Autodesk Inventor part; units mm, degrees
ref_plane "YZ Plane" through (0, 0, 0) normal (1, 0, 0) x (0, 1, 0)
ref_plane "XZ Plane" through (0, 0, 0) normal (0, 1, 0) x (-1, 0, 0)
ref_plane "XY Plane" through (0, 0, 0) normal (0, 0, 1) x (1, 0, 0)
sketch "Sketch1" plane through (0, 0, 0) normal (0, 0, 1) x (1, 0, 0)
  line L0 (-110, -113.5) -> (110, -113.5)
  line L1 (110, -113.5) -> (110, 113.5)
  line L2 (110, 113.5) -> (-110, 113.5)
  line L3 (-110, 113.5) -> (-110, -113.5)
  line L4 (-110, -113.5) -> (110, 113.5) construction
  line L5 (110, -113.5) -> (-110, 113.5) construction
  point P0 (0, 0)
  dimension "d0" = 220
  dimension "d1" = 227
extrude "Extrusion1" add sketch "Sketch1" along normal blind 8
sketch "Sketch2" plane through (0, 0, 8) normal (0, 0, 1) x (1, 0, 0)
  line L0 (-107.55, -111.05) -> (107.55, -111.05)
  line L1 (107.55, -111.05) -> (107.55, 111.05)
  line L2 (107.55, 111.05) -> (-107.55, 111.05)
  line L3 (-107.55, 111.05) -> (-107.55, -111.05)
  line L4 (-107.55, -111.05) -> (107.55, 111.05) construction
  line L5 (107.55, -111.05) -> (-107.55, 111.05) construction
  point P0 (0, 0)
  dimension "d4" = 215.1
  dimension "d5" = 222.1
extrude "Extrusion2" cut sketch "Sketch2" against normal blind 1.6
sketch "Sketch3" plane through (0, 0, 6.4) normal (0, 0, 1) x (1, 0, 0)
  line L0 (-105, -108.5) -> (105, -108.5)
  line L1 (105, -108.5) -> (105, 108.5)
  line L2 (105, 108.5) -> (-105, 108.5)
  line L3 (-105, 108.5) -> (-105, -108.5)
  line L4 (-105, -108.5) -> (105, 108.5) construction
  line L5 (105, -108.5) -> (-105, 108.5) construction
  point P0 (0, 0)
  dimension "d8" = 210
  dimension "d9" = 217
extrude "Extrusion3" cut sketch "Sketch3" against normal blind 3.5
fillet "Fillet1" radius 2 8 edges at (-107.55, -111.05, 7.2) (-110, -113.5, 4) (110, -113.5, 4) (107.55, -111.05, 7.2) (110, 113.5, 4) (107.55, 111.05, 7.2) (-110, 113.5, 4) (-107.55, 111.05, 7.2)
sketch "Sketch4" plane through (0, 0, 2.9) normal (0, 0, 1) x (1, 0, 0)
  circle A0 centre (-103.9, 107.4) radius 5
  circle A1 centre (-103.9, -107.4) radius 5
  line L0 (-105.55, 111.05) -> (105.55, 111.05)
  circle A2 centre (103.9, 107.4) radius 5
  line L1 (107.55, 109.05) -> (107.55, -109.05)
  circle A3 centre (103.9, -107.4) radius 5
  line L2 (-107.55, -109.05) -> (-107.55, 109.05)
  point P0 (0, 0)
  dimension "d13" = 10
  dimension "d14" = 10
  dimension "d15" = 214.8
  dimension "d16" = 3.65
  dimension "d17" = 10
  dimension "d18" = 207.8
  dimension "d19" = 3.65
  dimension "d20" = 10
  dimension "d21" = 3.65
  dimension "d22" = 214.8
  dimension "d23" = 207.8
  dimension "d24" = 3.65
extrude "Extrusion4" add sketch "Sketch4" along normal blind 3.5
sketch "Sketch5" plane through (0, 0, 6.4) normal (0, 0, 1) x (1, 0, 0)
  arc A0 (-105, 102.5225) -> (-99.0225, 108.5) centre (-103.9, 107.4) ccw
  circle A1 centre (-103.9, 107.4) radius 1.4
  arc A2 (99.0225, 108.5) -> (105, 102.5225) centre (103.9, 107.4) ccw
  circle A3 centre (103.9, 107.4) radius 1.4
  arc A4 (105, -102.5225) -> (99.0225, -108.5) centre (103.9, -107.4) ccw
  circle A5 centre (103.9, -107.4) radius 1.4
  arc A6 (-99.0225, -108.5) -> (-105, -102.5225) centre (-103.9, -107.4) ccw
  circle A7 centre (-103.9, -107.4) radius 1.4
  point P0 (0, 0)
  dimension "d27" = 2.8
  dimension "d28" = 2.8
  dimension "d29" = 2.8
  dimension "d30" = 2.8
extrude "Extrusion5" cut sketch "Sketch5" against normal blind 3.5
sketch "Sketch6" plane through (0, 0, 2.9) normal (0, 0, 1) x (1, 0, 0)
  circle A0 centre (0, -59.795) radius 8
  line L0 (105.55, -111.05) -> (-105.55, -111.05)
  circle A1 centre (0, 41.85) radius 8
  line L1 (-105.55, 111.05) -> (105.55, 111.05)
  circle A2 centre (0, -42.5) radius 8
  circle A3 centre (0, -20) radius 8
  circle A4 centre (0, 2.5) radius 8
  circle A5 centre (0, 25) radius 8
  point P0 (0, 0)
  dimension "d33" = 16
  dimension "d34" = 51.255
  dimension "d35" = 16
  dimension "d36" = 69.2
  dimension "d37" = 16
  dimension "d38" = 68.55
  dimension "d39" = 16
  dimension "d40" = 16
  dimension "d41" = 16
  dimension "d42" = 22.5
  dimension "d43" = 22.5
  dimension "d44" = 22.5
extrude "Extrusion6" add sketch "Sketch6" along normal blind 3.5
sketch "Sketch7" plane through (0, 41.85, 6.4) normal (0, 0, 1) x (1, 0, 0)
  circle A0 centre (0, 0) radius 8
  circle A1 centre (0, 0) radius 2.1
  circle A2 centre (0, -16.85) radius 8
  circle A3 centre (0, -16.85) radius 6
  circle A4 centre (0, -39.35) radius 8
  circle A5 centre (0, -39.35) radius 6
  circle A6 centre (0, -61.85) radius 8
  circle A7 centre (0, -61.85) radius 6
  circle A8 centre (0, -84.35) radius 8
  circle A9 centre (0, -84.35) radius 6
  circle A10 centre (0, -101.645) radius 8
  circle A11 centre (0, -101.645) radius 2.1
  point P0 (0, -41.85)
  dimension "d47" = 4.2
  dimension "d48" = 12
  dimension "d49" = 12
  dimension "d50" = 12
  dimension "d51" = 12
  dimension "d52" = 4.2
extrude "Extrusion7" cut sketch "Sketch7" against normal through all contours A1 | A3 | A5 | A7 | A9 | A11
properties part number "BasePlate"
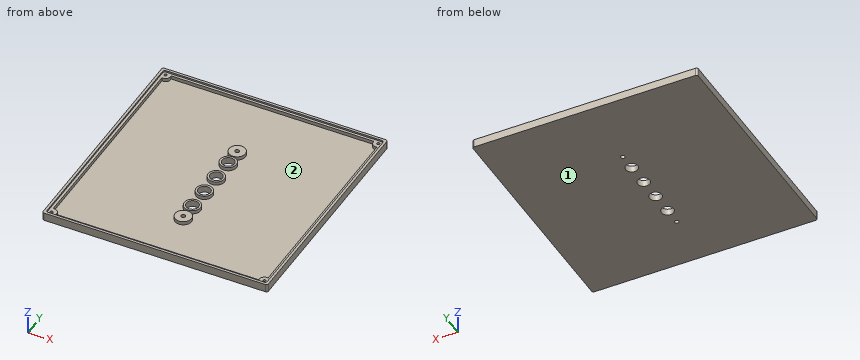
Part model, mm, in its own coordinate system. Face numbers are marked on the shaded views. Coordinates: 2 decimals unless noted, no trailing zeros. Loops run counter-clockwise (first coordinate to the right, second up) from the corner with the lowest first, then second, coordinate; pieces in that order, holes last. Notation, with made-up numbers: M 70.25,54 L 127.25,54 A14 ccw 127.25,74 Z; hole C 45,20.5 d4. An arc over 180 degrees is marked long. Use a Markdown table: item, result. Add a question column.
Q1. Mould opens along Y. For the marked faces 1 and 2 say: +Y half, -Y half, draft (parallel to the pull), parting line (faces both ways), or undercut.
Q2. Probe L1, parallel to X at y = -107.4, z = 5.75; L2, parallel to Y at x = -25.5, z = 5.5; L3, parallel to Y at x = 103.9, z = 3.7. List the from-to ranges inside material, lowest first.
Q3. Cut at C-C (y = -82.5). Write the cut outline in (x, z), and give its area (3 significant figures).
Q4. Cut at B-B (x = 91.5). Write the cut outline in (y, z), and give its area (3 significant figures).
Q5. Pin check, flat tips, straight feed: P1, Ø2, axis at x = 103.5, y = -108, coming from the +Z side; P2, Ø11, axis at x = 0, y = 25, coming from the -Z side; P3, Ø1.5, axis at x = -23, y = -16.5, coming from the +Z side. Stop position of each tip, or through.
Q6. Cut at A-A (y = 25). Write the cut outline in (x, z), and give its area (3 significant figures).
Worked out:
| question | item | result |
|---|---|---|
| 1 | face 1 | draft |
| 1 | face 2 | undercut |
| 2 | L1 | x = -110 to -105.3, -102.5 to -98.9, 98.9 to 102.5, 105.3 to 110 |
| 2 | L2 | y = -113.5 to -108.5, 108.5 to 113.5 |
| 2 | L3 | y = -113.5 to -108.8, -106 to -102.4, 102.4 to 106, 108.8 to 113.5 |
| 3 | outline | M -110,0 L 110,0 L 110,8 L 107.55,8 L 107.55,6.4 L 105,6.4 L 105,2.9 L -105,2.9 L -105,6.4 L -107.55,6.4 L -107.55,8 L -110,8 Z |
| 3 | area | 681 mm2 |
| 4 | outline | M -113.5,0 L 113.5,0 L 113.5,8 L 111.05,8 L 111.05,6.4 L 108.5,6.4 L 108.5,2.9 L -108.5,2.9 L -108.5,6.4 L -111.05,6.4 L -111.05,8 L -113.5,8 Z |
| 4 | area | 701 mm2 |
| 5 | P1 | stops at z = 6.4 |
| 5 | P2 | passes through |
| 5 | P3 | stops at z = 2.9 |
| 6 | outline | M -110,0 L -6,0 L -6,6.4 L -8,6.4 L -8,2.9 L -105,2.9 L -105,6.4 L -107.55,6.4 L -107.55,8 L -110,8 Z; M 6,0 L 110,0 L 110,8 L 107.55,8 L 107.55,6.4 L 105,6.4 L 105,2.9 L 8,2.9 L 8,6.4 L 6,6.4 Z |
| 6 | area | 660 mm2 |
